The model under review builds one solid part; all positions refer to its coordinate system, in mm. Face numbers are marked on the shaded views. A direction names the side the tool comes from. Round coordinates to 2 decimals unless told otherwise and drop trailing zeros. Loops run counter-clockwise (first coordinate to the right, second up) from the corner with the lowest first, then second, coordinate; pieces in that order, holes last. Notation, with made-up numbers: (-21, 25.5) -> (-1, 25.5) arc R27 cw to (-1, 59.5) -> close; hole circle Ø5 at (65, -14). An arc over 180 degrees is marked (long way). Use a Markdown table: item, result. Add a question column.
1) Consider section C-C on y = 4. Give the boundary of the cut face in (x, z).
2) Insertion check: pin 1 (1.8 mm diameter, centred on x = -7.75, y = 13.42, fed in from -Z); pin 2 (5 mm diameter, centred on x = -7.75, y = -13.42, fed in from -Z); pin 3 (6 mm diameter, centred on x = 10, z = -4, fed in from +Y); pin 4 (0.8 mm diameter, centred on y = 3.5, z = 1, fed in from +X). Each pin has a flat end and moves straight along its axis. Give the tip position at first contact, or say it passes through.
3) For the marked faces 1 and 2, list the 3-axis set-ups (+Z, -Z, +X, -X, +Y, -Y) from which the entire face can be reached by the end or side of a thin tool; tool diameter is ignored.
4) Wall thickness on probe 1 along Z at (x, y) = (-15, -25); probe 2 along X at (y, z) = (-25, -6); probe 3 along Z at (x, y) = (3.5, -22.5): over which ranges is each line inside the solid? List them lowest first.
5) Consider section A-A on z = -30.5. Give the boundary of the cut face in (x, y), plus the area to 3 significant figures.
6) Consider section D-D on x = 7.75. Give the boundary of the cut face in (y, z).
7) Consider section B-B on x = 0. Give the boundary of the cut face in (y, z), plus the area to 4 significant figures.
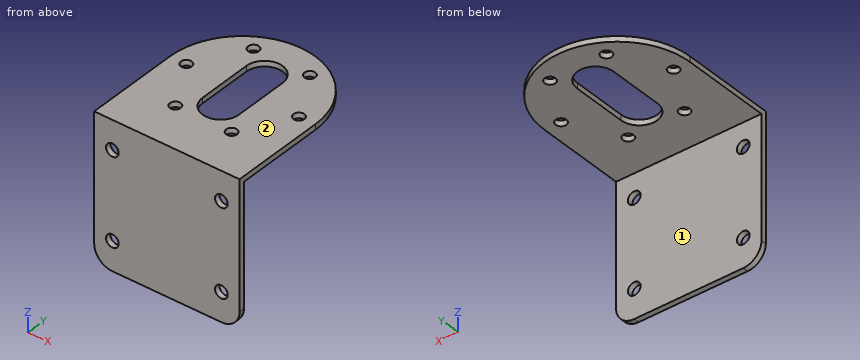
from build123d import *

# Parameters (mm, degrees)
SKETCH_1_R          = 1.5
EXTRUDE_1_DEPTH     = 1.5
SKETCH_2_W          = 40
SKETCH_2_H          = 1.5
EXTRUDE_2_DEPTH     = 38.5
SKETCH_3_R          = 1.75
CUT_EXTRUDE_1_DEPTH = 47
FILLET_1_R          = 5


with BuildPart() as part:
    # 草图1 → 凸台-拉伸1 (new body)
    with BuildSketch(Plane.XY):
        with BuildLine():
            Line((-20, 0), (-20, -26))
            Line((-20, -26), (20, -26))
            Line((20, -26), (20, 0))
            ThreePointArc((20, 0), (0, 20), (-20, 0))
        make_face()
        with Locations((7.75, 13.423393759)):
            Circle(SKETCH_1_R, mode=Mode.SUBTRACT)
        with Locations((-7.75, 13.423393759)):
            Circle(SKETCH_1_R, mode=Mode.SUBTRACT)
        with Locations((-15.5, 0)):
            Circle(SKETCH_1_R, mode=Mode.SUBTRACT)
        with Locations((-7.75, -13.423393759)):
            Circle(SKETCH_1_R, mode=Mode.SUBTRACT)
        with Locations((7.75, -13.423393759)):
            Circle(SKETCH_1_R, mode=Mode.SUBTRACT)
        with Locations((15.5, 0)):
            Circle(SKETCH_1_R, mode=Mode.SUBTRACT)
        with BuildLine():
            Line((5, -7.5), (5, 7.5))
            ThreePointArc((5, 7.5), (0, 12.5), (-5, 7.5))
            Line((-5, 7.5), (-5, -7.5))
            ThreePointArc((-5, -7.5), (0, -12.5), (5, -7.5))
        make_face(mode=Mode.SUBTRACT)
    extrude(amount=EXTRUDE_1_DEPTH)

    # 草图2 → 凸台-拉伸2 (add)
    with BuildSketch(Plane(origin=(0, 0, 0), x_dir=(-1, 0, 0), z_dir=(0, 0, -1))):
        with Locations((0, -25.25)):
            Rectangle(SKETCH_2_W, SKETCH_2_H)
    extrude(amount=EXTRUDE_2_DEPTH)

    # 草图3 → 切除-拉伸1 (cut, through all)
    with BuildSketch(Plane.XZ.offset(26)):
        with Locations((-15, -6.5)):
            Circle(SKETCH_3_R)
        with Locations((15, -6.5)):
            Circle(SKETCH_3_R)
        with Locations((-15, -30.5)):
            Circle(SKETCH_3_R)
        with Locations((15, -30.5)):
            Circle(SKETCH_3_R)
    extrude(amount=-CUT_EXTRUDE_1_DEPTH, mode=Mode.SUBTRACT)

    # 圆角1
    fillet_1_edges = [part.edges().sort_by_distance(p)[0] for p in [
        (20, -25.25, -38.5),
        (-20, -25.25, -38.5),
    ]]
    fillet(fillet_1_edges, radius=FILLET_1_R)


solid = part.part
Result set:
| question | item | result |
|---|---|---|
| 1 | outline | (-19.6, 0) -> (-5, 0) -> (-5, 1.5) -> (-19.6, 1.5) -> close; (5, 0) -> (19.6, 0) -> (19.6, 1.5) -> (5, 1.5) -> close |
| 2 | pin 1 | through |
| 2 | pin 2 | z = 0 |
| 2 | pin 3 | y = -24.5 |
| 2 | pin 4 | x = 19.76 |
| 3 | face 1 | -Z, +X, -X, +Y |
| 3 | face 2 | +Z, +X, -X, +Y, -Y |
| 4 | probe 1 | -38.5 to -32.25, -28.75 to -8.25, -4.75 to 1.5 |
| 4 | probe 2 | -20 to -16.68, -13.32 to 13.32, 16.68 to 20 |
| 4 | probe 3 | 0 to 1.5 |
| 5 | outline | (-20, -26) -> (-16.75, -26) -> (-16.75, -24.5) -> (-20, -24.5) -> close; (-13.25, -26) -> (13.25, -26) -> (13.25, -24.5) -> (-13.25, -24.5) -> close; (16.75, -26) -> (20, -26) -> (20, -24.5) -> (16.75, -24.5) -> close |
| 5 | area | 49.5 mm2 |
| 6 | outline | (-26, -38.5) -> (-24.5, -38.5) -> (-24.5, 0) -> (-14.92, 0) -> (-14.92, 1.5) -> (-26, 1.5) -> close; (-11.92, 0) -> (11.92, 0) -> (11.92, 1.5) -> (-11.92, 1.5) -> close; (14.92, 0) -> (18.44, 0) -> (18.44, 1.5) -> (14.92, 1.5) -> close |
| 7 | outline | (-26, -38.5) -> (-24.5, -38.5) -> (-24.5, 0) -> (-12.5, 0) -> (-12.5, 1.5) -> (-26, 1.5) -> close; (12.5, 0) -> (20, 0) -> (20, 1.5) -> (12.5, 1.5) -> close |
| 7 | area | 89.25 mm2 |
